Could you check a few things on this drawing? It's one solid part, dimensions in mm from its lowest x, y, z. A direction names the side the tool comes from. Give positions to 0.01 mm unless a question says otherwise; leave off trailing zeros. Order: outer loops, then holes, each group sorted by start corner. A loop starts at its lowest first (then second) coordinate and runs counter-clockwise, first axis right, second up. Notation, with made-up numbers: (89, 69) -> (94, 69) arc R16 ccw to (94, 79) -> close; hole circle Ø6 at (-19, 14). An arc over 180 degrees is marked (long way). Write each question's results on one line, items separated by ' | '. Start each with the question number.
Q1. I need wall thicknesses on line 1 along X through (y, z) = (1, 4) (3 decimals); line 2 along X through (y, z) = (4, 2.5) (1 decimal); line 3 along X through (y, z) = (0.5, 5.5) (3 decimals). Which ranges of each line are inside material? Lowest first, please. Write a range as [from, to].
Q2. For the marked faces 4, 5 and 6, which set-ups out of +Z, -Z, +X, -X, +Y, -Y let a thin tool reach every point of the face, with its end or its side?
Q3. Imagine slicing it at B-B, the plane x = 16. Please give me the cut outline in (y, z).
Q4. Imagine slicing it at D-D, the plane y = 1. Please give me the cut outline in (x, z) (3 decimals).
Q5. I'm going to push flat-ended pins straight in: pin 1 (1 mm diameter, centred on y = 7.5, z = 5, fed in from -X); pin 2 (4 mm diameter, centred on x = 29.5, z = 4.5, fed in from +Y). Where does each tip first touch, or does it pass through?
Q6. Imagine slicing it at A-A, the plane z = 4. State how many separate pieces and enclosed holes the cut face has, then the cut area to 3 significant figures.
Q7. Thinking about a two-plate mould opening in X: for the marked faces 1, 2 and 3, which applies, pulls with the +X half, pulls with the -X half, needs draft (parallel to the pull), parting line crosses it, or undercut?
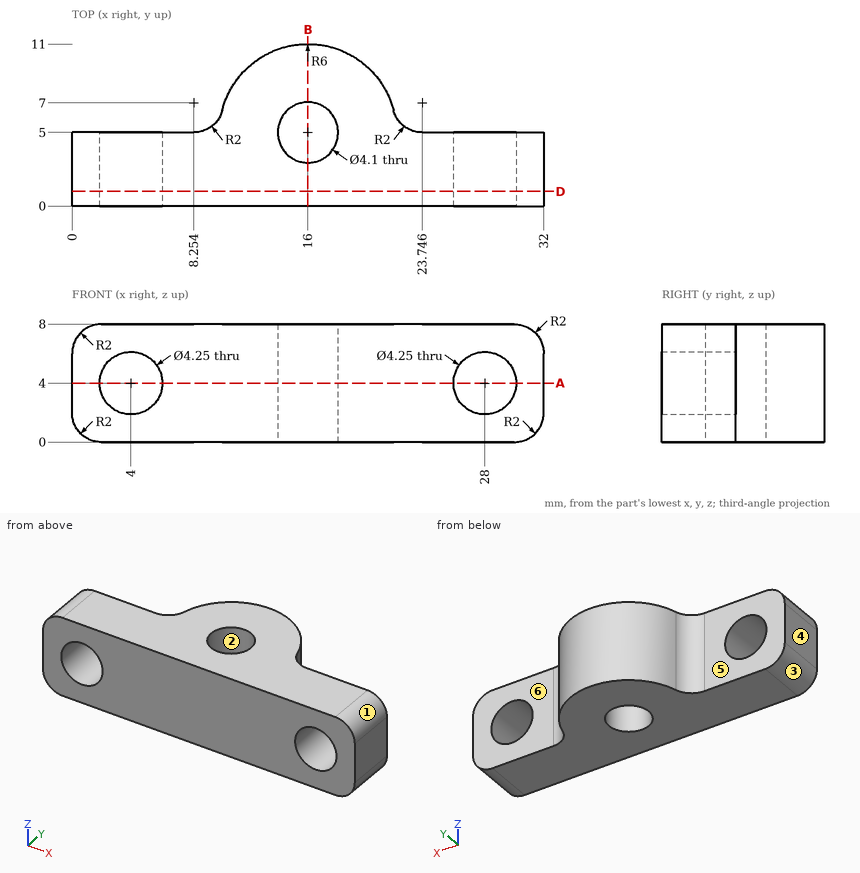
Geometry check:
1) line 1: [0, 1.875], [6.125, 25.875], [30.125, 32] | line 2: [0, 2.5], [5.5, 14.2], [17.8, 26.5], [29.5, 32] | line 3: [0, 2.495], [5.505, 26.495], [29.505, 32]
2) face 4: +Z, -Z, -X, +Y, -Y | face 5: +Z, -Z, -X, +Y | face 6: +Z, -Z, +X, +Y
3) outline: (0, 0) -> (2.95, 0) -> (2.95, 8) -> (0, 8) -> close; (7.05, 0) -> (11, 0) -> (11, 8) -> (7.05, 8) -> close
4) outline: (0, 2) arc R2 ccw to (2, 0) -> (30, 0) arc R2 ccw to (32, 2) -> (32, 6) arc R2 ccw to (30, 8) -> (2, 8) arc R2 ccw to (0, 6) -> close; hole circle Ø4.25 at (4, 4); hole circle Ø4.25 at (28, 4)
5) pin 1: x = 10.34 | pin 2: y = 5
6) separate pieces: 3 | enclosed holes: 1 | area: 162 mm²
7) face 1: pulls with the +X half | face 2: undercut | face 3: pulls with the -X half
